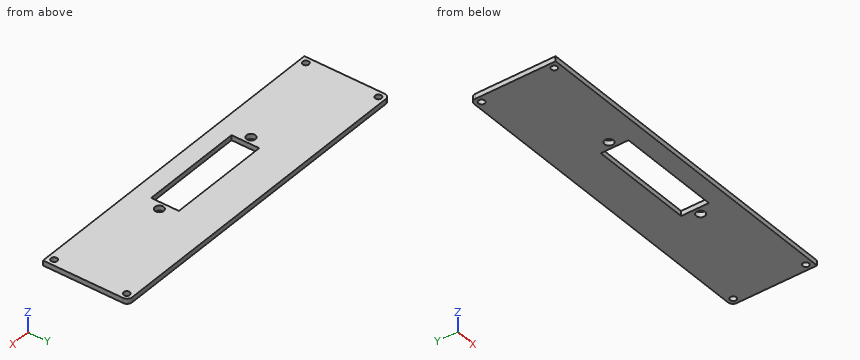
from build123d import *

# Parameters (mm, degrees)
SKETCH_W           = 134
SKETCH_H           = 33.8
PAD_DEPTH          = 2
SKETCH001_R        = 1.75
POCKET_DEPTH       = 2.001
FILLET_R           = 2
SKETCH002_R        = 1.25
POCKET001_DEPTH    = 278.424154
POLARPATTERN_COUNT = 2
SKETCH003_W        = 41.2
SKETCH003_H        = 11
POCKET002_DEPTH    = 5


with BuildPart() as part:
    # Sketch → Pad (new body)
    with BuildSketch(Plane.XY):
        Rectangle(SKETCH_W, SKETCH_H)
    extrude(amount=PAD_DEPTH)

    # Sketch001 (on Face6 of Pad) → Pocket (cut, through all)
    with BuildSketch(Plane.XY.offset(2)):
        with Locations((-23.5, -4.4)):
            Circle(SKETCH001_R)
        with Locations((23.5, -4.4)):
            Circle(SKETCH001_R)
    extrude(amount=-POCKET_DEPTH, mode=Mode.SUBTRACT)

    # Fillet
    fillet_edges = [part.edges().sort_by_distance(p)[0] for p in [
        (-67, 16.9, 1),
        (67, 16.9, 1),
    ]]
    fillet(fillet_edges, radius=FILLET_R)

    # Sketch002 → Pocket001 (cut, through all)
    with BuildSketch(Plane.XY):
        with Locations((-64.5, -14.4)):
            Circle(SKETCH002_R)
    pocket001 = extrude(amount=POCKET001_DEPTH, mode=Mode.SUBTRACT)

    # Mirrored: Pocket001 across YZ
    add(pocket001.mirror(Plane.YZ), mode=Mode.SUBTRACT)

    # Mirrored001: Pocket001 across XZ
    add(pocket001.mirror(Plane.XZ), mode=Mode.SUBTRACT)

    # PolarPattern: Pocket001 ×2 about axis
    polarpattern_axis = Axis((0, 0, 0), (0, 0, 1))
    for i in range(1, POLARPATTERN_COUNT):
        add(pocket001.rotate(polarpattern_axis, i * 360 / POLARPATTERN_COUNT), mode=Mode.SUBTRACT)

    # Sketch003 (on Face2 of PolarPattern) → Pocket002 (cut)
    with BuildSketch(Plane(origin=(0, 0, 0), x_dir=(1, 0, 0), z_dir=(0, 0, -1))):
        with Locations((0, 4.4)):
            Rectangle(SKETCH003_W, SKETCH003_H)
    extrude(amount=-POCKET002_DEPTH, mode=Mode.SUBTRACT)


solid = part.part
Verification items for the finished model (mm, model axes). Give positions to 0.01 mm unless a question says otherwise; leave off trailing zeros. Write each loop counter-clockwise with the first axis right and the second up, starting at its lowest first coordinate (ties: lowest second). Pieces come first, ordered by that corner, then holes. Notation, with made-up numbers: M 33,63 L 42,63 A15 ccw 42,85 Z; hole C -0.75,-36 d8. An arc over 180 degrees is marked long. Use CSV: the item, a comma, the result in double quotes.
1) Go/stop test with a flat-tipped pin: pin 1 Ø3 at (x, y) = (23.5, -4.4) entering from -Z. Record where the tip stops, or that it passes through.
Final values:
pin 1,"through"
2) Cross-section at B-B (x = 9). Enter the section's corners in (y, z), plus the area to 3 significant figures.
Final values:
outline,"M -16.9,0 L -9.9,0 L -9.9,2 L -16.9,2 Z; M 1.1,0 L 16.9,0 L 16.9,2 L 1.1,2 Z"
area,"45.6 mm²"
3) Cross-section at C-C (z = 0.8). Enter the section's corners in (x, y).
Final values:
outline,"M -67,-16.9 L 67,-16.9 L 67,14.9 A2 ccw 65,16.9 L -65,16.9 A2 ccw -67,14.9 Z; hole C -64.5,-14.4 d2.5; hole C -64.5,14.4 d2.5; hole C -23.5,-4.4 d3.5; hole M -20.6,-9.9 L 20.6,-9.9 L 20.6,1.1 L -20.6,1.1 Z; hole C 23.5,-4.4 d3.5; hole C 64.5,-14.4 d2.5; hole C 64.5,14.4 d2.5"
4) Cross-section at A-A (y = -0.5). Enter the section's corners in (x, z).
Final values:
outline,"M -67,0 L -20.6,0 L -20.6,2 L -67,2 Z; M 20.6,0 L 67,0 L 67,2 L 20.6,2 Z"
5) Material ranges on line 1 along Y through (x, z) = (64.5, 0.95); line 2 along Y through (x, z) = (23.5, 1); line 3 along Y through (x, z) = (19.5, 1.25), recorded low to high.
Final values:
line 1,"-16.9 to -15.65, -13.15 to 13.15, 15.65 to 16.9"
line 2,"-16.9 to -6.15, -2.65 to 16.9"
line 3,"-16.9 to -9.9, 1.1 to 16.9"
6) Cross-section at D-D (y = -14.4). Enter the section's corners in (x, z), plus the area to 3 significant figures.
Final values:
outline,"M -67,0 L -65.75,0 L -65.75,2 L -67,2 Z; M -63.25,0 L 63.25,0 L 63.25,2 L -63.25,2 Z; M 65.75,0 L 67,0 L 67,2 L 65.75,2 Z"
area,"258 mm²"
